Build history of the part. All positions in model axes, mm. A direction names the side the tool comes from. Coordinates: 2 decimals unless noted, no trailing zeros. Order: outer loops, then holes, each group sorted by start corner. A loop starts at its lowest first (then second) coordinate and runs counter-clockwise, first axis right, second up. Notation, with made-up numbers: M 54,75.25 L 103,75.25 A28 ccw 103,114.25 Z; hole C -18.5,18.25 d8. An arc over 180 degrees is marked long. Write item = value, one per line. Start each with the question number.
Q1. Drill centre lines: probe 1 along Y at (x, z) = (0, 43.5); probe 2 along Y at (x, z) = (0, 33); probe 3 along Y at (x, z) = (-11.5, 26). Where is each one in solid material? Low to high.
Q2. Pin check, flat tips, straight feed: P1, Ø13.5, axis at x = 5.5, y = 4.5, coming from the +Z side; P2, Ø3, axis at x = -10.5, z = 10, coming from the +Y side; P3, Ø3, axis at y = 14.5, z = 28, coming from the -X side; P4, Ø1.2, axis at y = 1, z = 16, coming from the -X side. Stop position of each tip, or through.
Q3. Band-saw the part on B-B on z = 14. Write the cut outline in (x, y).
Q4. Band-saw the part on D-D on z = 39.5. Write the cut outline in (x, y).
Q5. Band-saw the part on C-C on y = 3. Write the cut outline in (x, z), plus the area to 3 significant figures.
Q6. Band-saw the part on A-A on x = 0. Write the cut outline in (y, z), plus the area to 3 significant figures.
Q7. 3-axis set-ups, long thin cutter, end or side, ignore diameter. For faces 1 (the face through (6, -3, 23)), 2 (the face through (7, -2.05, 11)): which of +Z, -Z, +X, -X, +Y, -Y reach the whole face in a straight line?
```python
from build123d import *

# Parameters (mm, degrees)
F0_R     = 23
F3_DEPTH = 50
F4_R     = 13.5
F1_DEPTH = 27
F5_R     = 2.5
F2_DEPTH = 15


with BuildPart() as f3:
    # F0 (on Top) → F3 (new body)
    with BuildSketch(Plane.XY):
        Circle(F0_R)
        with BuildLine():
            ThreePointArc((-5.6921, 2.05), (0, 6.05), (5.6921, 2.05))
            Line((5.6921, 2.05), (8.1, 2.05))
            Line((8.1, 2.05), (8.1, -2.05))
            Line((8.1, -2.05), (5.6921, -2.05))
            ThreePointArc((5.6921, -2.05), (0, -6.05), (-5.6921, -2.05))
            Line((-5.6921, -2.05), (-8.1, -2.05))
            Line((-8.1, -2.05), (-8.1, 2.05))
            Line((-8.1, 2.05), (-5.6921, 2.05))
        make_face(mode=Mode.SUBTRACT)
        with BuildLine():
            ThreePointArc((-5.6921, -2.05), (-6.05, 0), (-5.6921, 2.05))
            Line((-5.6921, 2.05), (-8.1, 2.05))
            Line((-8.1, 2.05), (-8.1, -2.05))
            Line((-8.1, -2.05), (-5.6921, -2.05))
        make_face()
    extrude(amount=F3_DEPTH)

    # F4 (on face) → F1 (cut)
    with BuildSketch(Plane.XY.offset(50)):
        Circle(F4_R)
    extrude(amount=-F1_DEPTH, mode=Mode.SUBTRACT)

    # F5 (on face) → F2 (cut)
    with BuildSketch(Plane.XY.offset(50)):
        with Locations((15.588457, 9)):
            Circle(F5_R)
        with Locations((0, 18)):
            Circle(F5_R)
        with Locations((-15.588457, 9)):
            Circle(F5_R)
        with Locations((15.588457, -9)):
            Circle(F5_R)
        with Locations((0, -18)):
            Circle(F5_R)
        with Locations((-15.588457, -9)):
            Circle(F5_R)
    extrude(amount=-F2_DEPTH, mode=Mode.SUBTRACT)


solid = f3.part
```
Recorded:
q1.probe_1 = -23 to -20.5, -15.5 to -13.5, 13.5 to 15.5, 20.5 to 23
q1.probe_2 = -23 to -13.5, 13.5 to 23
q1.probe_3 = -19.92 to -7.07, 7.07 to 19.92
q2.P1 = 50
q2.P2 = 21.17
q2.P3 = -18.97
q2.P4 = -23
q3.outline = C 0,0 d46; hole M -5.69,-2.05 A6.05 ccw 5.69,-2.05 L 8.1,-2.05 L 8.1,2.05 L 5.69,2.05 A6.05 ccw -5.69,2.05 A6.05 ccw Z
q4.outline = C 0,0 d46; hole C -15.59,-9 d5; hole C -15.59,9 d5; hole C 0,0 d27; hole C 0,-18 d5; hole C 0,18 d5; hole C 15.59,-9 d5; hole C 15.59,9 d5
q5.outline = M -22.8,0 L -5.25,0 L -5.25,23 L -13.16,23 L -13.16,50 L -22.8,50 Z; M 5.25,0 L 22.8,0 L 22.8,50 L 13.16,50 L 13.16,23 L 5.25,23 Z
q5.area = 1,330 mm2
q6.outline = M -23,0 L -6.05,0 L -6.05,23 L -13.5,23 L -13.5,50 L -15.5,50 L -15.5,35 L -20.5,35 L -20.5,50 L -23,50 Z; M 6.05,0 L 23,0 L 23,50 L 20.5,50 L 20.5,35 L 15.5,35 L 15.5,50 L 13.5,50 L 13.5,23 L 6.05,23 Z
q6.area = 1,140 mm2
q7.face_1 = +Z
q7.face_2 = +Z, -Z
